The figure shows three views and two pictorial views of one solid part (mm, origin at its lowest corner). Answer the questions. A direction names the side the tool comes from. Give positions to 0.01 mm unless a question says otherwise; leave off trailing zeros. Loops run counter-clockwise (first coordinate to the right, second up) from the corner with the lowest first, then second, coordinate; pieces in that order, holes last. Notation, with made-up numbers: (47.25, 57.5) - (75.25, 57.5) arc R18 cw to (75.25, 77.5) - close; hole circle Ø8 at (77, -34). An arc over 180 degrees is marked (long way). One line per question, with ' | ' between items.
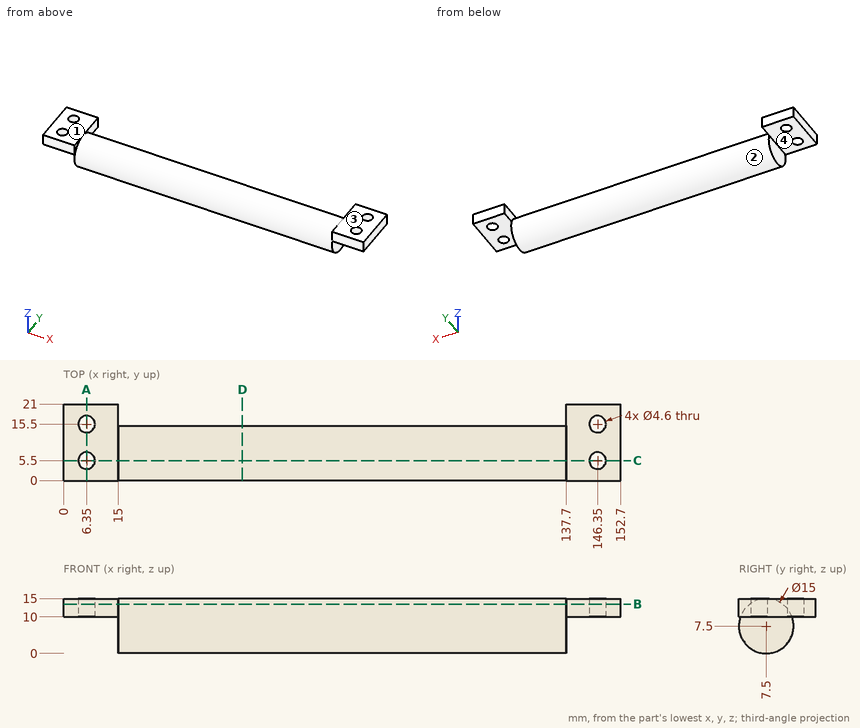
1. Find section A-A on x = 6.35. Write down the section's boundary in (y, z).
Evaluation:
outline: (0, 10) - (3.2, 10) - (3.2, 15) - (0, 15) - close; (7.8, 10) - (13.2, 10) - (13.2, 15) - (7.8, 15) - close; (17.8, 10) - (21, 10) - (21, 15) - (17.8, 15) - close
2. Which of the six approach directions +Z, -Z, +X, -X, +Y, -Y give full straight-line access (tool end or side, diameter ignored) to the marked faces 3 and 4?
Evaluation:
face 3: +Z, +X, -X, +Y, -Y | face 4: -Z, -X, +Y, -Y
3. Consider L1, parallel to X at y = 5.75, z = 13.75; L2, parallel to Y at x = 6.35, z = 11.65; L3, parallel to Z at x = 10, y = 18.75. Determine where each line is inside the solid, lowest interval first.
Evaluation:
L1: 0 to 4.06, 8.64 to 144.06, 148.64 to 152.7 | L2: 0 to 3.2, 7.8 to 13.2, 17.8 to 21 | L3: 10 to 15
4. Flat-ended cylindrical pins translate along their axes: pin 1 (2 mm diameter, centred on x = 40, z = 8.5, fed in from +Y); pin 2 (4.5 mm diameter, centred on x = 148, y = 13, fed in from -Z); pin 3 (8 mm diameter, centred on x = 133, z = 3, fed in from -Y). Find the tip coordinate at first contact, or state that the pin passes through.
Evaluation:
pin 1: y = 15 | pin 2: z = 10 | pin 3: y = 0.02
5. Find section B-B on z = 13.5. Write down the section's boundary in (x, y), then the cut area to 3 significant figures.
Evaluation:
outline: (0, 0) - (15, 0) - (15, 3) - (137.7, 3) - (137.7, 0) - (152.7, 0) - (152.7, 21) - (137.7, 21) - (137.7, 12) - (15, 12) - (15, 21) - (0, 21) - close; hole circle Ø4.6 at (6.35, 5.5); hole circle Ø4.6 at (6.35, 15.5); hole circle Ø4.6 at (146.35, 5.5); hole circle Ø4.6 at (146.35, 15.5) | area: 1,670 mm2
6. Find section C-C on y = 5.5. Write down the section's boundary in (x, z).
Evaluation:
outline: (0, 10) - (4.05, 10) - (4.05, 15) - (0, 15) - close; (8.65, 10) - (15, 10) - (15, 0.27) - (137.7, 0.27) - (137.7, 10) - (144.05, 10) - (144.05, 15) - (137.7, 15) - (137.7, 14.73) - (15, 14.73) - (15, 15) - (8.65, 15) - close; (148.65, 10) - (152.7, 10) - (152.7, 15) - (148.65, 15) - close
7. Find section D-D on x = 49. Write down the section's boundary in (y, z), then the cut area to 3 significant figures.
Evaluation:
outline: circle Ø15 at (7.5, 7.5) | area: 177 mm2
8. Determine the mould class of the marked faces 1 and 2 for opening direction X: +X half, -X half, draft (parallel to the pull), parting line (faces both ways), or undercut.
Evaluation:
face 1: draft | face 2: undercut
